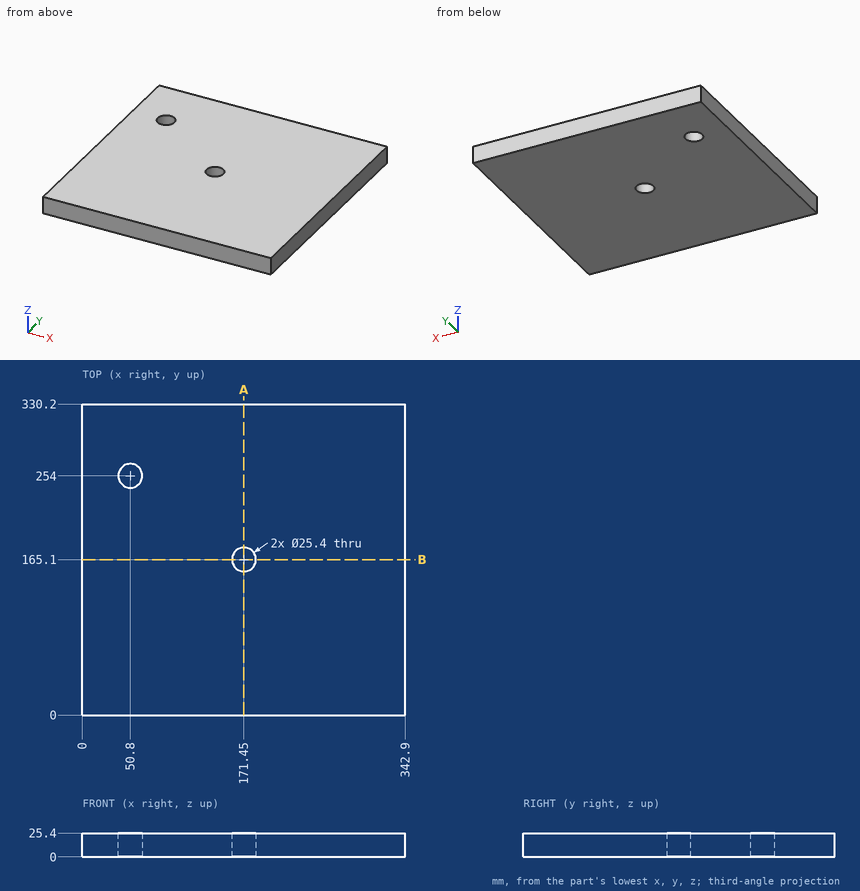
Check sheet for the drawn part. Datum: minimum x, y, z corner. Units: mm. Coordinates: 2 decimals unless noted, no trailing zeros. Loops run counter-clockwise (first coordinate to the right, second up) from the corner with the lowest first, then second, coordinate; pieces in that order, holes last. Notation, with made-up numbers: (17, -20.5) -> (61, -20.5) arc R14 ccw to (61, -6.5) -> close; hole circle Ø2 at (80.5, 56.25). An arc over 180 degrees is marked (long way). Answer in a Markdown table with one row per item.
1. Material ranges on line 1 along Y through (x, z) = (50.8, 14.25); line 2 along Y through (x, z) = (171.45, 11.75), recorded low to high. Write a range as [from, to].
Check values:
| item | result |
|---|---|
| line 1 | y = [0, 241.3], [266.7, 330.2] |
| line 2 | y = [0, 152.4], [177.8, 330.2] |
2. Go/stop test with a flat-tipped pin: pin 1 (8 mm diameter, centred on x = 290, y = 67.5, fed in from -Z). Record where the tip stops, or that it passes through.
Check values:
| item | result |
|---|---|
| pin 1 | stops at z = 0 |
3. Sectioned sample at A-A, the plane x = 171.45. Record the boundary of the cut face in (y, z), then the cut area to 3 significant figures.
Check values:
| item | result |
|---|---|
| outline | (0, 0) -> (152.4, 0) -> (152.4, 25.4) -> (0, 25.4) -> close; (177.8, 0) -> (330.2, 0) -> (330.2, 25.4) -> (177.8, 25.4) -> close |
| area | 7,740 mm2 |
4. Sectioned sample at B-B, the plane y = 165.1. Record the boundary of the cut face in (x, z), then the cut area to 3 significant figures.
Check values:
| item | result |
|---|---|
| outline | (0, 0) -> (158.75, 0) -> (158.75, 25.4) -> (0, 25.4) -> close; (184.15, 0) -> (342.9, 0) -> (342.9, 25.4) -> (184.15, 25.4) -> close |
| area | 8,060 mm2 |
